```python
from build123d import *

# Parameters (mm, degrees)
F0_W     = 50
F0_H     = 40
F1_DEPTH = 40
F2_W     = 44
F2_H     = 34
F3_DEPTH = 37
F4_R     = 3
F5_R     = 3


with BuildPart() as f1:
    # F0 (on Top) → F1 (new body)
    with BuildSketch(Plane.XY):
        with Locations((0, 20)):
            Rectangle(F0_W, F0_H)
    extrude(amount=F1_DEPTH)

    # F2 (on face) → F3 (cut)
    with BuildSketch(Plane.XY.offset(40)):
        with Locations((0, 20)):
            Rectangle(F2_W, F2_H)
    extrude(amount=-F3_DEPTH, mode=Mode.SUBTRACT)

    # F4
    f4_edges = [f1.edges().sort_by_distance(p)[0] for p in [
        (-22, 37, 21.5),
        (0, 37, 3),
        (-22, 20, 3),
        (-22, 3, 21.5),
        (0, 3, 3),
        (22, 20, 3),
        (22, 37, 21.5),
        (22, 3, 21.5),
    ]]
    fillet(f4_edges, radius=F4_R)

    # F5
    f5_edges = [f1.edges().sort_by_distance(p)[0] for p in [
        (-25, 0, 20),
        (25, 0, 20),
        (0, 0, 0),
        (-25, 20, 0),
        (-25, 40, 20),
        (0, 40, 0),
        (25, 20, 0),
        (25, 40, 20),
    ]]
    fillet(f5_edges, radius=F5_R)


solid = f1.part
```
Design review of the part built by this model. Coordinates are the model's own, in mm. A direction names the side the tool comes from. Round coordinates to 2 decimals unless told otherwise and drop trailing zeros. Write each loop counter-clockwise with the first axis right and the second up, starting at its lowest first coordinate (ties: lowest second). Pieces come first, ordered by that corner, then holes.
Item 1: For probe 1 along Y at (x, z) = (-18, 24.5); probe 2 along X at (y, z) = (19.5, 23.5); probe 3 along Z at (x, y) = (0.5, 7.5), list the stretches that pass through material, from the lowest coordinate up.
Item 2: The part is to be moulded in two halves that separate along X. For faces 1 (the cylindrical face through (-24.14, 39.1, 21.76)), 2 (the cylindrical face through (0.31, 0.86, 0.9)), 3 (the flat face through (0, 20, 3)), say which applies: +X half, -X half, draft (parallel to the pull), parting line (faces both ways), or undercut.
Item 3: We need section A-A on x = -8. Write out the cut boundary in (y, z).
Item 4: For faces 4 (the cylindrical face through (-21.1, 36.14, 22.76)), 5 (the cylindrical face through (24.14, 20.24, 0.9)), list the 3-axis set-ups (+Z, -Z, +X, -X, +Y, -Y) from which the entire face can be reached by the end or side of a thin tool; tool diameter is ignored.
Item 5: We need section C-C on y = 12. Write out the cut boundary in (x, z).
Item 6: Clearance check with a flat-ended pin moving along its axis: pin 1 Ø22.5 at (x, y) = (-3.5, 20.5) entering from +Z. State where the tip first meets the part, or that it passes through.
Item 7: We need section B-B on z = 29.5. Write out the cut boundary in (x, y), and give its area (3 significant figures).
Returned:
1. probe 1: y = 0 to 3, 37 to 40
1. probe 2: x = -25 to -22, 22 to 25
1. probe 3: z = 0 to 3
2. face 1: -X half
2. face 2: draft
2. face 3: undercut
3. outline: (0, 3) arc R3 ccw to (3, 0) - (37, 0) arc R3 ccw to (40, 3) - (40, 40) - (37, 40) - (37, 6) arc R3 cw to (34, 3) - (6, 3) arc R3 cw to (3, 6) - (3, 40) - (0, 40) - close
4. face 4: +Z
4. face 5: -Z, +X, +Y, -Y
5. outline: (-25, 3) arc R3 ccw to (-22, 0) - (22, 0) arc R3 ccw to (25, 3) - (25, 40) - (22, 40) - (22, 6) arc R3 cw to (19, 3) - (-19, 3) arc R3 cw to (-22, 6) - (-22, 40) - (-25, 40) - close
6. pin 1: stops at z = 3
7. outline: (-25, 3) arc R3 ccw to (-22, 0) - (22, 0) arc R3 ccw to (25, 3) - (25, 37) arc R3 ccw to (22, 40) - (-22, 40) arc R3 ccw to (-25, 37) - close; hole (-22, 6) arc R3 ccw to (-19, 3) - (19, 3) arc R3 ccw to (22, 6) - (22, 34) arc R3 ccw to (19, 37) - (-19, 37) arc R3 ccw to (-22, 34) - close
7. area: 504 mm2
